from build123d import *

# Parameters (mm, degrees)
F0_W           = 600
F0_H           = 2000
F1_DEPTH       = 400
F2_T           = -20
F4_DEPTH       = 70
F5_W           = 25
F5_H           = 30
F6_DEPTH       = 12.5
F7_W           = 300
F7_H           = 44.7851331079
F7_W_2         = 45
F7_W_3         = 255
F7_H_2         = 175.2148668921
F8_DEPTH       = 1000
F8_DEPTH_BACK  = 950
F10_R          = 27.9824593268
F11_DEPTH      = 600.001
F11_DEPTH_BACK = 600.001


with BuildPart() as f1:
    # F0 (on Top) → F1 (new body)
    with BuildSketch(Plane.XY):
        with Locations((-300, 0)):
            Rectangle(F0_W, F0_H)
    extrude(amount=F1_DEPTH)

    # F2
    f2_openings = [f1.faces().sort_by_distance(p)[0] for p in [
        (-300, 0, 400),
        (0, 0, 200),
    ]]
    offset(amount=F2_T, openings=f2_openings)

    # F3 (on face) → F4 (join)
    with BuildSketch(Plane.XZ.offset(1000)):
        with BuildLine():
            Line((0, 18.4187632612), (0, 256.5082568117))
            ThreePointArc((0, 256.5082568117), (-119.0447467752, 137.4635100365), (0, 18.4187632612))
        make_face()
        with BuildLine():
            ThreePointArc((0, 18.4187632612), (84.1773477094, 53.2861623271), (119.0447467752, 137.4635100365))
            ThreePointArc((119.0447467752, 137.4635100365), (84.1773477094, 221.6408577459), (0, 256.5082568117))
            Line((0, 256.5082568117), (0, 18.4187632612))
        make_face()
    extrude(amount=F4_DEPTH)

    # F5 (on Right) → F6 (join, symmetric)
    with BuildSketch(Plane.YZ):
        with Locations((900, 15)):
            Rectangle(F5_W, F5_H)
        with BuildLine():
            ThreePointArc((912.5, 30), (900, 42.5), (887.5, 30))
            Line((887.5, 30), (912.5, 30))
        make_face()
    extrude(amount=F6_DEPTH, both=True)

    # F7 (on Front) → F8 (join, two sides)
    with BuildSketch(Plane.XZ) as f8_sk:
        with Locations((-150, -22.392566554)):
            Rectangle(F7_W, F7_H)
        with Locations((-322.5, -22.392566554)):
            Rectangle(F7_W_2, F7_H)
        with Locations((-472.5, -22.392566554)):
            Rectangle(F7_W_3, F7_H)
        with Locations((-322.5, -132.392566554)):
            Rectangle(F7_W_2, F7_H_2)
    extrude(amount=F8_DEPTH)
    extrude(f8_sk.sketch, amount=-F8_DEPTH_BACK)

    # F9: F1 across plane


with BuildPart() as f1_1:
    add(f1.part)
    add(f1.part.mirror(Plane.YZ))

    # F10 (on Right) → F11 (cut, two sides)
    with BuildSketch(Plane.YZ) as f11_sk:
        with Locations((500, -130.9047937393)):
            Circle(F10_R)
    extrude(amount=-F11_DEPTH, mode=Mode.SUBTRACT)
    extrude(f11_sk.sketch, amount=F11_DEPTH_BACK, mode=Mode.SUBTRACT)


solid = f1_1.part
Verification items for the finished model (mm, model axes). A direction names the side the tool comes from. Give positions to 0.01 mm unless a question says otherwise; leave off trailing zeros. Write each loop counter-clockwise with the first axis right and the second up, starting at its lowest first coordinate (ties: lowest second). Pieces come first, ordered by that corner, then holes.
(1) Material ranges on line 1 (X direction, y = 604, z = -174); line 2 (Y direction, x = 440.5, z = 214); line 3 (Z direction, x = 333, y = 500), recorded low to high.
(2) Cross-section at A-A (y = -131). Enter the section's corners in (x, z).
(3) Cross-section at C-C (x = 424). Enter the section's corners in (y, z), plus the area to 3 significant figures.
(4) Mould release check, pull along X, two halves, no side actions. Record for faces 1 (the face through (8, 975, 0)), 2 (the face through (-345, -39, -134)), 3 (the face through (300, -39, -134)): +X half, -X half, draft (parallel to the pull), parting line (faces both ways), or undercut.
(5) Cross-section at D-D (z = 81.5). Enter the section's corners in (x, y).
(6) Access from +Z, -Z, +X, -X, +Y, -Y to the whole of each face (thin tool, end or side, straight path). Record for faces 4 (the face through (-300, -39, -134)), 5 (the face through (474, -39, -44.785)), 6 (the face through (600, -14, 174)), 7 (the face through (-2, -1070, 139)), 8 (the face through (8, 980, 207)).
(7) Cross-section at B-B (z = 341). Enter the section's corners in (x, y), plus the area to 3 significant figures.
(8) Gauge pin test, flat ends, axial feed: pin 1 (4 mm diameter, centred on x = 453, z = 245.5, fed in from -Y); pin 2 (2 mm diameter, centred on y = 65, z = -100, fed in from +X); pin 3 (3 mm diameter, centred on x = -213, y = -134, fed in from +Z). Record the tip position at first contact, or that the pin passes through.
Worked out:
1. line 1: x = -345 to -300, 300 to 345
1. line 2: y = -1000 to -980, 980 to 1000
1. line 3: z = -220 to -158.89, -102.92 to 20
2. outline: (-600, -44.79) - (-345, -44.79) - (-345, -220) - (-300, -220) - (-300, -44.79) - (300, -44.79) - (300, -220) - (345, -220) - (345, -44.79) - (600, -44.79) - (600, 400) - (580, 400) - (580, 20) - (-580, 20) - (-580, 400) - (-600, 400) - close
3. outline: (-1000, -44.79) - (950, -44.79) - (950, 0) - (1000, 0) - (1000, 400) - (980, 400) - (980, 20) - (-980, 20) - (-980, 400) - (-1000, 400) - close
3. area: 143,000 mm2
4. face 1: draft
4. face 2: -X half
4. face 3: undercut
5. outline: (-600, -1000) - (-105.07, -1000) - (-105.07, -1070) - (105.07, -1070) - (105.07, -1000) - (600, -1000) - (600, 1000) - (-600, 1000) - close; hole (-580, -980) - (580, -980) - (580, 980) - (-580, 980) - close
6. face 4: -Z, +Y, -Y
6. face 5: -Z, +X, +Y, -Y
6. face 6: +Z, -Z, +X, +Y, -Y
6. face 7: +Z, -Z, +X, -X, -Y
6. face 8: +Z
7. outline: (-600, -1000) - (600, -1000) - (600, 1000) - (-600, 1000) - close; hole (-580, -980) - (580, -980) - (580, 980) - (-580, 980) - close
7. area: 126,000 mm2
8. pin 1: stops at y = -1000
8. pin 2: stops at x = 345
8. pin 3: stops at z = 20
